Geometry check sheet. Reference: the model listing, model coordinates, mm. A direction names the side the tool comes from. Round coordinates to 2 decimals unless told otherwise and drop trailing zeros. Write each loop counter-clockwise with the first axis right and the second up, starting at its lowest first coordinate (ties: lowest second). Pieces come first, ordered by that corner, then holes. Notation, with made-up numbers: M -14,44 L -6,44 A16 ccw -6,68 Z; hole C 45.5,41.5 d2. An arc over 180 degrees is marked long. Answer in a Markdown table with one row per item. Add a question column.
from build123d import *

# Parameters (mm, degrees)
MODEL_R                  = 1.5
MODEL_R_2                = 2
RESSALTO_EXTRUS_O1_DEPTH = 15
ESBO_O1_R                = 2.5
CORTE_EXTRUS_O1_DEPTH    = 10
ESBO_O2_R                = 2.5
CORTE_EXTRUS_O2_DEPTH    = 10
CHANFRO1_SIZE            = 2.5


with BuildPart() as part:
    # Model → Ressalto-extrusão1 (new body)
    with BuildSketch(Plane.XY):
        with BuildLine():
            Line((45.959420932, 55.536238099), (45.959420932, 415.536238099))
            ThreePointArc((45.959420932, 415.536238099), (47.423887026, 419.071772005), (50.959420932, 420.536238099))
            Line((50.959420932, 420.536238099), (410.959420932, 420.536238099))
            ThreePointArc((410.959420932, 420.536238099), (414.494954838, 419.071772005), (415.959420932, 415.536238099))
            Line((415.959420932, 415.536238099), (415.959420932, 55.536238099))
            ThreePointArc((415.959420932, 55.536238099), (414.494954838, 52.000704193), (410.959420932, 50.536238099))
            Line((410.959420932, 50.536238099), (390.959420932, 50.536238099))
            Line((390.959420932, 50.536238099), (388.959420932, 52.536238099))
            Line((388.959420932, 52.536238099), (384.959420932, 56.536238099))
            Line((384.959420932, 56.536238099), (378.959420932, 56.536238099))
            Line((378.959420932, 56.536238099), (374.959420932, 52.536238099))
            Line((374.959420932, 52.536238099), (86.959420932, 52.536238099))
            Line((86.959420932, 52.536238099), (82.959420932, 56.536238099))
            Line((82.959420932, 56.536238099), (76.959420932, 56.536238099))
            Line((76.959420932, 56.536238099), (72.959420932, 52.536238099))
            Line((72.959420932, 52.536238099), (70.959420932, 50.536238099))
            Line((70.959420932, 50.536238099), (50.959420932, 50.536238099))
            ThreePointArc((50.959420932, 50.536238099), (47.423887026, 52.000704193), (45.959420932, 55.536238099))
        make_face()
        with Locations((95.959420932, 56.536238099)):
            Circle(MODEL_R, mode=Mode.SUBTRACT)
        with Locations((365.959420932, 56.536238099)):
            Circle(MODEL_R, mode=Mode.SUBTRACT)
        with Locations((275.959420932, 56.536238099)):
            Circle(MODEL_R, mode=Mode.SUBTRACT)
        with Locations((185.959420932, 56.536238099)):
            Circle(MODEL_R, mode=Mode.SUBTRACT)
        with Locations((55.959420932, 90.536238099)):
            Circle(MODEL_R, mode=Mode.SUBTRACT)
        with Locations((75.959420932, 90.536238099)):
            Circle(MODEL_R, mode=Mode.SUBTRACT)
        with Locations((65.959420932, 70.536238099)):
            Circle(MODEL_R, mode=Mode.SUBTRACT)
        with Locations((395.959420932, 70.536238099)):
            Circle(MODEL_R, mode=Mode.SUBTRACT)
        with Locations((385.959420932, 90.536238099)):
            Circle(MODEL_R, mode=Mode.SUBTRACT)
        with Locations((405.959420932, 90.536238099)):
            Circle(MODEL_R, mode=Mode.SUBTRACT)
        with Locations((405.959420932, 410.536238099)):
            Circle(MODEL_R, mode=Mode.SUBTRACT)
        with Locations((385.959420932, 410.536238099)):
            Circle(MODEL_R, mode=Mode.SUBTRACT)
        with Locations((55.959420932, 410.536238099)):
            Circle(MODEL_R, mode=Mode.SUBTRACT)
        with Locations((75.959420932, 410.536238099)):
            Circle(MODEL_R, mode=Mode.SUBTRACT)
        with Locations((93.910965405, 118.501571518)):
            Circle(MODEL_R, mode=Mode.SUBTRACT)
        with Locations((50.910965405, 212.501571518)):
            Circle(MODEL_R, mode=Mode.SUBTRACT)
        with Locations((93.910965405, 212.501571518)):
            Circle(MODEL_R, mode=Mode.SUBTRACT)
        with Locations((50.876198806, 118.527793034)):
            Circle(MODEL_R, mode=Mode.SUBTRACT)
        with Locations((95.959420932, 63.536238099)):
            Circle(MODEL_R, mode=Mode.SUBTRACT)
        with Locations((365.959420932, 63.536238099)):
            Circle(MODEL_R, mode=Mode.SUBTRACT)
        with Locations((275.959420932, 63.536238099)):
            Circle(MODEL_R, mode=Mode.SUBTRACT)
        with Locations((185.959420932, 63.536238099)):
            Circle(MODEL_R, mode=Mode.SUBTRACT)
        with Locations((84.709420932, 126.036238099)):
            Circle(MODEL_R, mode=Mode.SUBTRACT)
        with Locations((75.209420932, 126.036238099)):
            Circle(MODEL_R, mode=Mode.SUBTRACT)
        with Locations((374.959420932, 136.436238099)):
            Circle(MODEL_R_2, mode=Mode.SUBTRACT)
        with Locations((374.959420932, 286.436238099)):
            Circle(MODEL_R_2, mode=Mode.SUBTRACT)
        with BuildLine():
            Line((140.959420932, 67.536238099), (140.959420932, 82.536238099))
            Line((140.959420932, 82.536238099), (137.423887026, 86.071772005))
            ThreePointArc((137.423887026, 86.071772005), (135.801770282, 87.155635761), (133.88835312, 87.536238099))
            Line((133.88835312, 87.536238099), (105.959420932, 87.536238099))
            ThreePointArc((105.959420932, 87.536238099), (102.423887026, 89.000704193), (100.959420932, 92.536238099))
            Line((100.959420932, 92.536238099), (100.959420932, 375.536238099))
            ThreePointArc((100.959420932, 375.536238099), (102.423887026, 379.071772005), (105.959420932, 380.536238099))
            Line((105.959420932, 380.536238099), (355.959420932, 380.536238099))
            ThreePointArc((355.959420932, 380.536238099), (359.494954838, 379.071772005), (360.959420932, 375.536238099))
            Line((360.959420932, 375.536238099), (360.959420932, 92.536238099))
            ThreePointArc((360.959420932, 92.536238099), (359.494954838, 89.000704193), (355.959420932, 87.536238099))
            Line((355.959420932, 87.536238099), (328.030488744, 87.536238099))
            ThreePointArc((328.030488744, 87.536238099), (326.117071582, 87.155635761), (324.494954838, 86.071772005))
            Line((324.494954838, 86.071772005), (320.959420932, 82.536238099))
            Line((320.959420932, 82.536238099), (320.959420932, 67.536238099))
            ThreePointArc((320.959420932, 67.536238099), (315.959420932, 62.536238099), (310.959420932, 67.536238099))
            Line((310.959420932, 67.536238099), (310.959420932, 82.536238099))
            Line((310.959420932, 82.536238099), (307.423887026, 86.071772005))
            ThreePointArc((307.423887026, 86.071772005), (305.801770282, 87.155635761), (303.88835312, 87.536238099))
            Line((303.88835312, 87.536238099), (263.030488744, 87.536238099))
            ThreePointArc((263.030488744, 87.536238099), (261.117071582, 87.155635761), (259.494954838, 86.071772005))
            Line((259.494954838, 86.071772005), (237.423887026, 67.000704193))
            ThreePointArc((237.423887026, 67.000704193), (235.801770282, 65.916840436), (233.88835312, 65.536238099))
            Line((233.88835312, 65.536238099), (228.030488744, 65.536238099))
            ThreePointArc((228.030488744, 65.536238099), (226.117071582, 65.916840436), (224.494954838, 67.000704193))
            Line((224.494954838, 67.000704193), (202.423887026, 86.071772005))
            ThreePointArc((202.423887026, 86.071772005), (200.801770282, 87.155635761), (198.88835312, 87.536238099))
            Line((198.88835312, 87.536238099), (158.030488744, 87.536238099))
            ThreePointArc((158.030488744, 87.536238099), (156.117071582, 87.155635761), (154.494954838, 86.071772005))
            Line((154.494954838, 86.071772005), (150.959420932, 82.536238099))
            Line((150.959420932, 82.536238099), (150.959420932, 67.536238099))
            ThreePointArc((150.959420932, 67.536238099), (145.959420932, 62.536238099), (140.959420932, 67.536238099))
        make_face(mode=Mode.SUBTRACT)
    extrude(amount=RESSALTO_EXTRUS_O1_DEPTH)

    # Esboço1 → Corte-extrusão1 (cut)
    with BuildSketch(Plane(origin=(0, 0, 0), x_dir=(-1, 0, 0), z_dir=(0, 0, -1))):
        with Locations((-385.959420932, 90.536238099)):
            Circle(ESBO_O1_R)
        with Locations((-405.959420932, 90.536238099)):
            Circle(ESBO_O1_R)
        with Locations((-395.959420932, 70.536238099)):
            Circle(ESBO_O1_R)
        with Locations((-75.959420932, 90.536238099)):
            Circle(ESBO_O1_R)
        with Locations((-55.959420932, 90.536238099)):
            Circle(ESBO_O1_R)
        with Locations((-65.959420932, 70.536238099)):
            Circle(ESBO_O1_R)
        with Locations((-405.959420932, 410.536238099)):
            Circle(ESBO_O1_R)
        with Locations((-385.959420932, 410.536238099)):
            Circle(ESBO_O1_R)
        with Locations((-75.959420932, 410.536238099)):
            Circle(ESBO_O1_R)
        with Locations((-55.959420932, 410.536238099)):
            Circle(ESBO_O1_R)
        with Locations((-84.709420932, 126.036238099)):
            Circle(ESBO_O1_R)
        with Locations((-75.209420932, 126.036238099)):
            Circle(ESBO_O1_R)
    extrude(amount=-CORTE_EXTRUS_O1_DEPTH, mode=Mode.SUBTRACT)

    # Esboço2 → Corte-extrusão2 (cut)
    with BuildSketch(Plane.XY.offset(15)):
        with Locations((50.910965405, 212.501571518)):
            Circle(ESBO_O2_R)
        with Locations((93.910965405, 212.501571518)):
            Circle(ESBO_O2_R)
        with Locations((93.910965405, 118.501571518)):
            Circle(ESBO_O2_R)
        with Locations((50.876198806, 118.527793034)):
            Circle(ESBO_O2_R)
    extrude(amount=-CORTE_EXTRUS_O2_DEPTH, mode=Mode.SUBTRACT)

    # Chanfro1
    chanfro1_edges = [part.edges().sort_by_distance(p)[0] for p in [
        (372.959420932, 136.436238099, 15),
        (372.959420932, 286.436238099, 15),
    ]]
    chamfer(chanfro1_edges, length=CHANFRO1_SIZE)


solid = part.part
Item 1: Mould release check, pull along X, two halves, no side actions. Record for faces 4 (the flat face through (61, 50.536, 7)), 5 (the conical face through (376.919, 285.624, 12.621)): +X half, -X half, draft (parallel to the pull), parting line (faces both ways), or undercut.
Item 2: Access from +Z, -Z, +X, -X, +Y, -Y to the whole of each face (thin tool, end or side, straight path). Record for faces 1 (the flat face through (120, 87.536, 7)), 2 (the flat face through (233, 52.536, 7)), 3 (the flat face through (228, 420.536, 7)).
Item 3: Section check A-A, the plane x = 287. Record the boundary of the cut face in (y, z).
Item 4: Section check B-B, the plane y = 100. Record the boundary of the cut face in (x, z).
Item 5: Section check C-C, the plane z = 7.25. Give the number of separate pieces and of enclosed holes in the cut face, and give its area (3 significant figures).
Item 6: Gauge pin test, flat ends, axial feed: pin 1 Ø2.5 at (x, y) = (65.5, 71) entering from -Z; pin 2 Ø8 at (x, z) = (173, 4.5) entering from -Y; pin 3 Ø5 at (x, z) = (81, 10) entering from -Y. Record the tip position at first contact, or that the pin passes through.
Item 7: Scan lines: probe 1 along X at (y, z) = (172, 9.25); probe 2 along Y at (x, z) = (179.5, 13.75); probe 3 along X at (y, z) = (285, 3). Record each from-to range of solid material in increasing order. Write a range as from..to.
Result sheet:
| question | item | result |
|---|---|---|
| 1 | face 4 | draft |
| 1 | face 5 | undercut |
| 2 | face 1 | +Z, -Z |
| 2 | face 2 | +Z, -Z, -Y |
| 2 | face 3 | +Z, -Z, +X, -X, +Y |
| 3 | outline | M 52.54,0 L 87.54,0 L 87.54,15 L 52.54,15 Z; M 380.54,0 L 420.54,0 L 420.54,15 L 380.54,15 Z |
| 4 | outline | M 45.96,0 L 100.96,0 L 100.96,15 L 45.96,15 Z; M 360.96,0 L 415.96,0 L 415.96,15 L 360.96,15 Z |
| 5 | separate pieces | 1 |
| 5 | enclosed holes | 27 |
| 5 | area | 58,300 mm^2 |
| 6 | pin 1 | stops at z = 10 |
| 6 | pin 2 | stops at y = 52.54 |
| 6 | pin 3 | stops at y = 56 |
| 7 | probe 1 | x = 45.96..100.96, 360.96..415.96 |
| 7 | probe 2 | y = 52.54..87.54, 380.54..420.54 |
| 7 | probe 3 | x = 45.96..100.96, 360.96..373.57, 376.35..415.96 |
